Can you work these out from the model? Positions are in its coordinate system, mm. Give positions to 0.01 mm unless a question says otherwise; leave off trailing zeros. Order: outer loops, then holes, each group sorted by start corner. A loop starts at its lowest first (then second) coordinate and runs counter-clockwise, first axis right, second up. Notation, with made-up numbers: (43.5, -1) - (53.5, -1) arc R14 cw to (53.5, 9) - close; hole circle Ø6 at (76, 17.5). An arc over 180 degrees is marked (long way). Answer as CSV lines item,"result".
```python
from build123d import *

# Parameters (mm, degrees)
SKETCH_1_W      = 33.02
SKETCH_1_H      = 8.5
EXTRUDE_1_DEPTH = 2.5
SKETCH_2_W      = 0.6
SKETCH_2_H      = 0.4
EXTRUDE_2_DEPTH = 3


with BuildPart() as part:
    # Эскиз1 → Бобышка-Вытянуть1 (new body)
    with BuildSketch(Plane(origin=(0, 0, 0), x_dir=(1, 0, 0), z_dir=(0, 1, 0))):
        Rectangle(SKETCH_1_W, SKETCH_1_H)
    extrude(amount=EXTRUDE_1_DEPTH)

    # Эскиз2 → Бобышка-Вытянуть2 (add)
    with BuildSketch(Plane.XY.offset(4.25)):
        with Locations((-7.62, 1.25)):
            Rectangle(SKETCH_2_W, SKETCH_2_H)
        with Locations((-10.16, 1.25)):
            Rectangle(SKETCH_2_W, SKETCH_2_H)
        with Locations((-5.08, 1.25)):
            Rectangle(SKETCH_2_W, SKETCH_2_H)
        with Locations((-2.54, 1.25)):
            Rectangle(SKETCH_2_W, SKETCH_2_H)
        with Locations((0, 1.25)):
            Rectangle(SKETCH_2_W, SKETCH_2_H)
        with Locations((2.54, 1.25)):
            Rectangle(SKETCH_2_W, SKETCH_2_H)
        with Locations((5.08, 1.25)):
            Rectangle(SKETCH_2_W, SKETCH_2_H)
        with Locations((7.62, 1.25)):
            Rectangle(SKETCH_2_W, SKETCH_2_H)
        with Locations((10.180976984, 1.25)):
            Rectangle(SKETCH_2_W, SKETCH_2_H)
        with Locations((12.720976984, 1.25)):
            Rectangle(SKETCH_2_W, SKETCH_2_H)
        with Locations((15.260976984, 1.25)):
            Rectangle(SKETCH_2_W, SKETCH_2_H)
        with Locations((-12.7, 1.25)):
            Rectangle(SKETCH_2_W, SKETCH_2_H)
        with Locations((-15.24, 1.25)):
            Rectangle(SKETCH_2_W, SKETCH_2_H)
    extrude(amount=EXTRUDE_2_DEPTH)


solid = part.part
```
1) I need wall thicknesses on line 1 along Z through (x, y) = (-11, 0.35); line 2 along Y through (x, z) = (10, 5). Which ranges of each line are inside material? Lowest first, please. Write a range as [from, to].
Answer block:
line 1,"[-4.25, 4.25]"
line 2,"[1.05, 1.45]"
2) I want a section at B-B on y = 0.6. Write out the boundary of the cut face in (x, z), plus the area to 3 significant figures.
Answer block:
outline,"(-16.51, -4.25) - (16.51, -4.25) - (16.51, 4.25) - (-16.51, 4.25) - close"
area,"281 mm2"
3) I want a section at A-A on z = 6.25. Count the separate pieces of the cut face and the enclosed holes in it, plus the area to 3 significant figures.
Answer block:
separate pieces,"13"
enclosed holes,"0"
area,"3.12 mm2"
4) I want a section at C-C on x = 6.5. Write out the boundary of the cut face in (y, z), plus the area to 4 significant figures.
Answer block:
outline,"(0, -4.25) - (2.5, -4.25) - (2.5, 4.25) - (0, 4.25) - close"
area,"21.25 mm2"
5) I'm going to push flat-ended pins straight in: P1, Ø0.5, axis at x = -5, z = 5.5, coming from the -Y side; P2, Ø0.5, axis at x = 0, z = 6, coming from the +Y side. Where does each tip first touch, or does it pass through?
Answer block:
P1,"y = 1.05"
P2,"y = 1.45"
